from build123d import *

# Parameters (mm, degrees)
F0_R     = 16
F1_DEPTH = 21
F0_R_2   = 9
F2_DEPTH = 16
F3_R     = 16
F4_DEPTH = 4
F5_DEPTH = 16
F6_R     = 7
F0_R_3   = 4.2
F7_DEPTH = 5


with BuildPart() as f1:
    # F0 (on Front) → F1 (new body)
    with BuildSketch(Plane.XZ):
        Circle(F0_R)
        Polygon((-12.417059955, -7.1295129852), (-12.3828693393, 7.1887328687), (0.0341906157, 14.318245854), (12.417059955, 7.1295129852), (12.3828693393, -7.1887328687), (-0.0341906157, -14.318245854), align=None, mode=Mode.SUBTRACT)
    extrude(amount=F1_DEPTH)



with BuildPart() as f2:
    # F0 (on Front) → F2 (new body)
    with BuildSketch(Plane.XZ):
        Circle(F0_R_2)
        Polygon((-3.8840263382, -6.6240223986), (-7.6785848415, 0.0516542785), (-3.7945585034, 6.6756766771), (3.8840263382, 6.6240223986), (7.6785848415, -0.0516542785), (3.7945585034, -6.6756766771), align=None, mode=Mode.SUBTRACT)
    extrude(amount=F2_DEPTH)


with BuildPart() as f1_1:
    add(f1.part)

    add(f2.part)  # F4 merges F2
    # F3 (on Front) → F4 (join)
    with BuildSketch(Plane.XZ):
        Circle(F3_R)
    extrude(amount=-F4_DEPTH)

    # F0 (on Front) → F5 (join)
    with BuildSketch(Plane.XZ):
        Polygon((0.0341906157, 14.318245854), (-12.3828693393, 7.1887328687), (-12.417059955, -7.1295129852), (-0.0341906157, -14.318245854), (12.3828693393, -7.1887328687), (12.417059955, 7.1295129852), align=None)
        Circle(F0_R_2, mode=Mode.SUBTRACT)
    extrude(amount=F5_DEPTH)

    # F6
    f6_edges = [f1_1.edges().sort_by_distance(p)[0] for p in [
        (-16, 4, 0),
    ]]
    fillet(f6_edges, radius=F6_R)

    # F0 (on Front) → F7 (join)
    with BuildSketch(Plane.XZ):
        Polygon((-3.7945585034, 6.6756766771), (-7.6785848415, 0.0516542785), (-3.8840263382, -6.6240223986), (3.7945585034, -6.6756766771), (7.6785848415, -0.0516542785), (3.8840263382, 6.6240223986), align=None)
        Circle(F0_R_3, mode=Mode.SUBTRACT)
    extrude(amount=F7_DEPTH)


solid = f1_1.part
Build history of the part. All positions in model axes, mm. A direction names the side the tool comes from. Round coordinates to 2 decimals unless told otherwise and drop trailing zeros. Loops run counter-clockwise (first coordinate to the right, second up) from the corner with the lowest first, then second, coordinate; pieces in that order, holes last. Notation, with made-up numbers: (83, -14) -> (120, -14) arc R16 ccw to (120, -3) -> close; hole circle Ø7 at (10, 89). An arc over 180 degrees is marked (long way). Answer in a Markdown table with one row per item.
Item 1: Pin check, flat tips, straight feed: pin 1 (2 mm diameter, centred on x = 5.5, y = -6.5, fed in from +Z); pin 2 (1.5 mm diameter, centred on x = 11, z = 6.5, fed in from +Y); pin 3 (12.5 mm diameter, centred on x = -4.5, z = -5, fed in from -Y); pin 4 (2 mm diameter, centred on y = -15, z = -5, fed in from +X). Stop position of each tip, or through.
Answers below:
| item | result |
|---|---|
| pin 1 | stops at z = 15.35 |
| pin 2 | stops at y = 3.31 |
| pin 3 | stops at y = -21 |
| pin 4 | stops at x = 15.49 |
Item 2: Saw through at A-A (y = -15). Write the cut outline in (x, z).
Answers below:
| item | result |
|---|---|
| outline | circle Ø32 at (0, 0); hole (-7.68, 0.05) -> (-3.88, -6.62) -> (3.79, -6.68) -> (7.68, -0.05) -> (3.88, 6.62) -> (-3.79, 6.68) -> close |
Item 3: Drill centre lines: L1, parallel to Z at x = 0, y = -3.55; L2, parallel to Y at x = -0.5, z = 3.5; L3, parallel to X at y = -17.5, z = 4. Where is each one in solid material? Low to high. Write a range as [from, to].
Answers below:
| item | result |
|---|---|
| L1 | z = [-16, -4.2], [4.2, 16] |
| L2 | y = [0, 4] |
| L3 | x = [-15.49, -12.39], [12.41, 15.49] |
Item 4: Saw through at C-C (y = -1.25). Write the cut outline in (x, z).
Answers below:
| item | result |
|---|---|
| outline | circle Ø31.56 at (0, 0); hole circle Ø8.4 at (0, 0) |
Item 5: Which spindle directions (+Z, -Z, +X, -X, +Y, -Y) get a long thin tool onto all of the face, cutting with end or side? Do faces 4 (the flat face through (-5.76, -10.42, 3.32)), 5 (the flat face through (5, -21, -12)). Say none if no direction does.
Answers below:
| item | result |
|---|---|
| face 4 | -Y |
| face 5 | +Z, -Z, +X, -X, -Y |
Item 6: Saw through at B-B (y = -3.75). Write the cut outline in (x, z).
Answers below:
| item | result |
|---|---|
| outline | circle Ø32 at (0, 0); hole circle Ø8.4 at (0, 0) |
Item 7: Mould opens along X. For faces 1 (the flat face through (5.76, -10.42, -3.32)), 2 (the cylindrical face through (-3.47, -12.13, -15.62)), 3 (the flat face through (0, 4, 0)) say: +X half, -X half, draft (parallel to the pull), parting line (faces both ways), or undercut.
Answers below:
| item | result |
|---|---|
| face 1 | undercut |
| face 2 | parting line |
| face 3 | draft |
